Source: CAD feature listing. Evaluate the final solid. Frame: model axes, mm. Coordinates: 2 decimals unless noted, no trailing zeros. Order: outer loops, then holes, each group sorted by start corner. A loop starts at its lowest first (then second) coordinate and runs counter-clockwise, first axis right, second up.
```python
from build123d import *

# Parameters (mm, degrees)
SKETCH_R           = 20
PAD_DEPTH          = 20
PAD_TAPER          = 10
SKETCH001_R        = 2.5
POCKET_DEPTH       = 20
POCKET_TAPER       = -6
POLARPATTERN_COUNT = 15


with BuildPart() as part:
    # Sketch → Pad (new body)
    with BuildSketch(Plane.XY):
        Circle(SKETCH_R)
    extrude(amount=PAD_DEPTH, taper=PAD_TAPER)

    # Sketch001 → Pocket (cut)
    with BuildSketch(Plane.XY):
        with Locations((0, 20)):
            Circle(SKETCH001_R)
    pocket = extrude(amount=POCKET_DEPTH, taper=POCKET_TAPER, mode=Mode.SUBTRACT)

    # PolarPattern: Pocket ×15 about axis
    polarpattern_axis = Axis((0, 0, 0), (0, 0, 1))
    for i in range(1, POLARPATTERN_COUNT):
        add(pocket.rotate(polarpattern_axis, i * 360 / POLARPATTERN_COUNT), mode=Mode.SUBTRACT)


solid = part.part
```
1. Pin query (flat end, axial travel): P1, Ø1, axis at x = 3, z = 6.5, coming from the -Y side; P2, Ø8, axis at y = -2.5, z = 10.5, coming from the -X side; P3, Ø6, axis at x = 1.5, z = 17.5, coming from the +Y side. Return the tip coordinate at first contact, or that it passes through.
Findings:
P1: stops at y = -16.85
P2: stops at x = -18.46
P3: stops at y = 17.14
2. Ray query, line 1 (X direction, y = -17.5, z = 3.25); line 2 (X direction, y = 15, z = 11.25); line 3 (Y direction, x = -16, z = 16.5). Return the intervals inside material, ascending.
Findings:
line 1: x = -8.44 to -6.11, -2.2 to 2.2, 6.11 to 8.44
line 2: x = -9.98 to -9.83, -6.44 to 6.44, 9.83 to 9.98
line 3: y = -5.98 to -3.76, -0.42 to 3.21
3. Section query B-B on x = 0. Return loops of the section in (y, z), plus the area to 3 significant figures.
Findings:
outline: (-20, 0) - (17.5, 0) - (15.4, 20) - (-16.47, 20) - close
area: 694 mm2
4. Draft query along X for faces 1 (the face through (-17.327, -5.607, 10.14)), 2 (the face through (10.722, 14.721, 10.14)), 3 (the face through (3.5, -16.3, 7.9)). Return one class per face: released by +X, released by -X, zero draft, split by the parting line, or undercut.
Findings:
face 1: released by -X
face 2: released by +X
face 3: undercut
